```python
from build123d import *

# Parameters (mm, degrees)
ESQUISSE1_R                               = 14
BOSS_EXTRU_1_DEPTH                        = 150
CHANFREIN1_SIZE                           = 1
DIAM_TRE_DU_PER_AGE_14_0_14_1_D           = 14
DIAM_TRE_DU_PER_AGE_14_0_14_1_DEPTH       = 35
DIAM_TRE_DU_PER_AGE_14_0_14_1_CSINK_D     = 15
DIAM_TRE_DU_PER_AGE_14_0_14_1_CSINK_ANGLE = 90
DIAM_TRE_DU_PER_AGE_14_0_14_1_TIP         = 4.206024333
CHANFREIN2_SIZE                           = 0.5
TROU_TARAUD_M8X1_01_D                     = 7
TROU_TARAUD_M8X1_01_DEPTH                 = 25
TROU_TARAUD_M8X1_01_TIP                   = 2.103012167
ENL_V_MAT_EXTRU_1_REACH                   = 152
ESQUISSE13_W                              = 5.5
ESQUISSE13_H                              = 4.102839415
CHANFREIN3_SIZE                           = 1
CHANFREIN4_SIZE                           = 1


with BuildPart() as part:
    # Esquisse1 → Boss.-Extru.1 (new body)
    with BuildSketch(Plane(origin=(0, 0, 0), x_dir=(1, 0, 0), z_dir=(0, 1, 0))):
        with Locations(Location((0, 0, 0), (0, 0, 270))):  # turned: the seam where the file's is
            Circle(ESQUISSE1_R)
    extrude(amount=BOSS_EXTRU_1_DEPTH)

    # Chanfrein1
    chanfrein1_edges = [part.edges().sort_by_distance(p)[0] for p in [
        (0, 150, -14),
    ]]
    chamfer(chanfrein1_edges, length=CHANFREIN1_SIZE)

    # Diamètre du perçage Ø14.0 (14)1
    with Locations(Plane(origin=(0, 150, 0), x_dir=(-1, 0, 0), z_dir=(0, 1, 0))):
        with Locations((0, 0)):
            CounterSinkHole(DIAM_TRE_DU_PER_AGE_14_0_14_1_D / 2, DIAM_TRE_DU_PER_AGE_14_0_14_1_CSINK_D / 2, depth=DIAM_TRE_DU_PER_AGE_14_0_14_1_DEPTH, counter_sink_angle=DIAM_TRE_DU_PER_AGE_14_0_14_1_CSINK_ANGLE)
            with Locations((0, 0, -(DIAM_TRE_DU_PER_AGE_14_0_14_1_DEPTH + DIAM_TRE_DU_PER_AGE_14_0_14_1_TIP / 2))):  # 118° drill point
                Cone(0, DIAM_TRE_DU_PER_AGE_14_0_14_1_D / 2, DIAM_TRE_DU_PER_AGE_14_0_14_1_TIP, mode=Mode.SUBTRACT)

    # Chanfrein2
    chanfrein2_edges = [part.edges().sort_by_distance(p)[0] for p in [
        (0, 0, -14),
    ]]
    chamfer(chanfrein2_edges, length=CHANFREIN2_SIZE)

    # Trou taraudé M8x1.01
    with Locations(Plane.XZ):
        with Locations((0, 0)):
            Hole(TROU_TARAUD_M8X1_01_D / 2, depth=TROU_TARAUD_M8X1_01_DEPTH)
            with Locations((0, 0, -(TROU_TARAUD_M8X1_01_DEPTH + TROU_TARAUD_M8X1_01_TIP / 2))):  # 118° drill point
                Cone(0, TROU_TARAUD_M8X1_01_D / 2, TROU_TARAUD_M8X1_01_TIP, mode=Mode.SUBTRACT)

    # Esquisse11 → Trou taraudé M42 (revolve, cut)
    with BuildSketch(Plane(origin=(0, 140, 0), x_dir=(0, 1, 0), z_dir=(1, 0, 0))):
        Polygon((0, 0), (0, 14), (2.25, 14), (1.65, 13.4), (1.65, 0), align=None)
    revolve(axis=Axis((0, 140, -6.35), (0, 0, 1)), mode=Mode.SUBTRACT)

    # Esquisse13 → Enlèv. mat.-Extru.1 (cut, up to next)
    with BuildSketch(Plane(origin=(0, 150, 0), x_dir=(-1, 0, 0), z_dir=(0, 1, 0)), mode=Mode.PRIVATE) as enl_v_mat_extru_1_sk1:
        with Locations((0, -12.551419707)):
            Rectangle(ESQUISSE13_W, ESQUISSE13_H)
    enl_v_mat_extru_1_tool1 = extrude(enl_v_mat_extru_1_sk1.sketch, amount=-ENL_V_MAT_EXTRU_1_REACH, mode=Mode.PRIVATE) & part.part
    add(enl_v_mat_extru_1_tool1.solids().sort_by_distance((0, 150, -12.55142))[0], mode=Mode.SUBTRACT)

    # Chanfrein3
    chanfrein3_edges = [part.edges().sort_by_distance(p)[0] for p in [
        (2.75, 0, -11.858469944),
        (-2.75, 0, -11.858469944),
        (0, 0, -10.5),
    ]]
    chamfer(chanfrein3_edges, length=CHANFREIN3_SIZE)

    # Chanfrein4
    chanfrein4_edges = [part.edges().sort_by_distance(p)[0] for p in [
        (2.75, 150, -11.60290288),
        (-2.75, 150, -11.60290288),
        (0, 150, -10.5),
    ]]
    chamfer(chanfrein4_edges, length=CHANFREIN4_SIZE)


solid = part.part
```
Could you check a few things on this model? Use its own coordinates, in mm. A direction names the side the tool comes from. Round coordinates to 2 decimals unless told otherwise and drop trailing zeros. Write each loop counter-clockwise with the first axis right and the second up, starting at its lowest first coordinate (ties: lowest second). Pieces come first, ordered by that corner, then holes. Notation, with made-up numbers: M 77,-18.5 L 117,-18.5 A9 cw 117,-8.5 Z; hole C 36.5,61.5 d10. An arc over 180 degrees is marked long. Write each question's results on one line, items separated by ' | '. Start each with the question number.
1. On a 3-axis mill with a long thin cutter (end or side, diameter ignored), from which of +Z, -Z, +X, -X, +Y, -Y can I reach the whole of each face in a straight line? I mean faces 4 (the face through (-3.233, 12.675, -1.341)), 5 (the face through (-0.496, 141.574, 10.055)), 6 (the face through (-1.517, 132.008, -6.834)), 7 (the face through (-6, 150, 6)), 8 (the face through (-2.75, 76, -12)). Say none if no direction works.
2. I need wall thicknesses on L1, parallel to Z at x = 0, y = 130; L2, parallel to X at y = 14, z = 0; L3, parallel to Y at x = 0, z = 9.5. Which ranges of each line are inside material? Lowest first, please. Write a range as from..to.
3. Imagine slicing it at A-A on y = 125.5. List the corners of the cut face in (x, z) for me, and give its area (3 significant figures).
4. Thinking about a two-plate mould opening in X: for faces 1 (the face through (-0.54, 149.84, 13.15)), 2 (the face through (-3, 0, 3)), 3 (the face through (2.75, 76, -12)), which applies, +X half, -X half, draft (parallel to the pull), parting line (faces both ways), or undercut?
5. I'm going to push flat-ended pins straight in: pin 1 Ø6 at (y, z) = (85.5, 5) entering from +X; pin 2 Ø6.5 at (x, z) = (0, 0) entering from -Y; pin 3 Ø12 at (x, y) = (11, 48.5) entering from -Z. Where does each tip first touch, or does it pass through?
6. Imagine slicing it at C-C on y = 10. List the corners of the cut face in (x, z) for me.
7. Imagine slicing it at B-B on y = 33. List the corners of the cut face in (x, z) for me.
Result sheet:
1) face 4: -Y | face 5: +Z | face 6: +Y | face 7: +Z, -Z, +X, -X, +Y | face 8: -Z, +Y, -Y
2) L1: z = -10.5..-7, 7..14 | L2: x = -14..-3.5, 3.5..14 | L3: y = 0..138.35, 141.65..150
3) outline: M -2.75,-13.73 L -2.75,-10.5 L 2.75,-10.5 L 2.75,-13.73 A14 ccw long Z; hole C 0,0 d14 | area: 443 mm^2
4) face 1: parting line | face 2: draft | face 3: undercut
5) pin 1: stops at x = 13.86 | pin 2: stops at y = 25.15 | pin 3: stops at z = -13.08
6) outline: M -2.75,-13.73 L -2.75,-10.5 L 2.75,-10.5 L 2.75,-13.73 A14 ccw long Z; hole C 0,0 d7
7) outline: M -2.75,-13.73 L -2.75,-10.5 L 2.75,-10.5 L 2.75,-13.73 A14 ccw long Z
